Source: CAD feature listing. Evaluate the final solid. Frame: model axes, mm. Give positions to 0.01 mm unless a question says otherwise; leave off trailing zeros. Loops run counter-clockwise (first coordinate to the right, second up) from the corner with the lowest first, then second, coordinate; pieces in that order, holes last. Notation, with made-up numbers: M -6,34 L 11,34 A18 cw 11,41 Z; hole C 72,-24 d2. An arc over 180 degrees is marked long. Put each result on its own line as item: value.
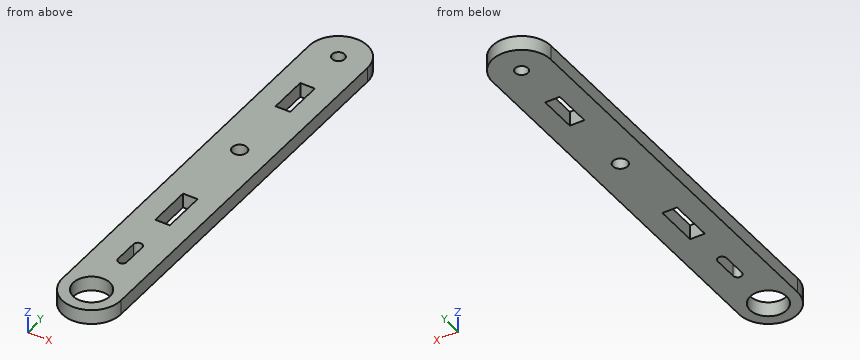
from build123d import *

# Parameters (mm, degrees)
MODEL_R             = 3.750000001
MODEL_R_2           = 1.300000002
MODEL_R_3           = 1.500000002
MODEL_W             = 3
MODEL_H             = 9
MODEL_H_2           = 8
BOSS_EXTRUDE1_DEPTH = 3


with BuildPart() as part:
    # Model → Boss-Extrude1 (new body)
    with BuildSketch(Plane.XY):
        with BuildLine():
            Line((56.05776, -3.869466211), (56.05776, 76.130633789))
            ThreePointArc((56.05776, 76.130633789), (62.05781, 82.130583788), (68.05776, 76.130533788))
            Line((68.05776, 76.130533788), (68.05776, -3.869466211))
            ThreePointArc((68.05776, -3.869466211), (62.057759999, -9.869466211), (56.05776, -3.869466211))
        make_face()
        with Locations((62.057759999, -3.869466212)):
            Circle(MODEL_R, mode=Mode.SUBTRACT)
        with Locations((62.057759998, 76.130533787)):
            Circle(MODEL_R_2, mode=Mode.SUBTRACT)
        with Locations((62.057760002, 44.130633787)):
            Circle(MODEL_R_3, mode=Mode.SUBTRACT)
        with BuildLine():
            Line((61.15776, 11.130633789), (61.15776, 6.130533789))
            ThreePointArc((61.15776, 6.130533789), (62.05776, 5.230533789), (62.95776, 6.130533789))
            Line((62.95776, 6.130533789), (62.95776, 11.130533786))
            ThreePointArc((62.95776, 11.130533786), (62.057810001, 12.030583787), (61.15776, 11.130633789))
        make_face(mode=Mode.SUBTRACT)
        with Locations((62.05776, 23.630533789)):
            Rectangle(MODEL_W, MODEL_H, mode=Mode.SUBTRACT)
        with Locations((62.05776, 62.130533789)):
            Rectangle(MODEL_W, MODEL_H_2, mode=Mode.SUBTRACT)
    extrude(amount=BOSS_EXTRUDE1_DEPTH)


solid = part.part
1. Section query A-A (y = 65). Output: boundary loops of the cut face in (x, z).
Found:
outline: M 56.06,0 L 60.56,0 L 60.56,3 L 56.06,3 Z; M 63.56,0 L 68.06,0 L 68.06,3 L 63.56,3 Z
2. Section query C-C (x = 57). Output: boundary loops of the cut face in (y, z), plus the area to 3 significant figures.
Found:
outline: M -7.1,0 L 79.36,0 L 79.36,3 L -7.1,3 Z
area: 259 mm^2
3. Section query B-B (z = 0.5). Output: boundary loops of the cut face in (x, y), plus the area to 3 significant figures.
Found:
outline: M 56.06,-3.87 A6 ccw 68.06,-3.87 L 68.06,76.13 A6 ccw 56.06,76.13 Z; hole C 62.06,-3.87 d7.5; hole M 60.56,19.13 L 63.56,19.13 L 63.56,28.13 L 60.56,28.13 Z; hole C 62.06,44.13 d3; hole M 60.56,58.13 L 63.56,58.13 L 63.56,66.13 L 60.56,66.13 Z; hole C 62.06,76.13 d2.6; hole M 61.16,6.13 A0.9 ccw 62.96,6.13 L 62.96,11.13 A0.9 ccw 61.16,11.13 Z
area: 954 mm^2
4. Material intervals for line 1 (X direction, y = 62, z = 1.4); line 2 (Y direction, x = 59.25, z = 2.4); line 3 (X direction, y = 44.5, z = 1.7), sorted ascending. Write a range as from..to.
Found:
line 1: 56.06..60.56, 63.56..68.06
line 2: -9.17..-6.36, -1.38..81.43
line 3: 56.06..60.6, 63.51..68.06
